from build123d import *

# Parameters (mm, degrees)
F2_START = 1.5
F0_W     = 68
F0_H     = 32
F0_W_2   = 66.0000007396
F0_H_2   = 30
F2_DEPTH = 4.5
F5_START = 0.9
F3_W     = 9.7086578608
F3_H     = 13.6771607213
F5_DEPTH = 2.3
F6_START = 1
F1_W     = 13.5039854795
F1_H     = 7.9890675843
F1_W_2   = 10.1785697043
F1_W_3   = 10.0000035018
F1_H_2   = 7.8571438789
F6_DEPTH = 4.6
F7_START = 1.5
F4_W     = 54.7266360372
F4_H     = 8.1930877641
F7_DEPTH = 4


with BuildPart() as f2:
    # F0 (on Top) → F2 (new body)
    with BuildSketch(Plane.XY.offset(F2_START)):
        with Locations((0, -0.0852976367)):
            Rectangle(F0_W, F0_H)
        with Locations((0, -0.0852976367)):
            Rectangle(F0_W_2, F0_H_2, mode=Mode.SUBTRACT)
    extrude(amount=F2_DEPTH)

    # F3 (on Top) → F5 (cut)
    with BuildSketch(Plane.XY.offset(F5_START)):
        with Locations((-30.4173231125, 1.8361529801)):
            Rectangle(F3_W, F3_H)
    extrude(amount=F5_DEPTH, mode=Mode.SUBTRACT)

    # F1 (on Top) → F6 (cut)
    with BuildSketch(Plane.XY.offset(F6_START)):
        with Locations((-19.5872941986, -13.5481059551)):
            Rectangle(F1_W, F1_H)
        with Locations((8.9285718277, -13.5481059551)):
            Rectangle(F1_W_2, F1_H)
        with Locations((21.8750005588, -13.4821441025)):
            Rectangle(F1_W_3, F1_H_2)
    extrude(amount=F6_DEPTH, mode=Mode.SUBTRACT)

    # F4 (on Top) → F7 (cut)
    with BuildSketch(Plane.XY.offset(F7_START)):
        with Locations((0.0114953145, 13.3686042391)):
            Rectangle(F4_W, F4_H)
    extrude(amount=F7_DEPTH, mode=Mode.SUBTRACT)


solid = f2.part
Read the model definition and answer for the solid it produces. Units are mm, in the model's axes. A direction names the side the tool comes from. Round coordinates to 2 decimals unless told otherwise and drop trailing zeros. Write each loop counter-clockwise with the first axis right and the second up, starting at its lowest first coordinate (ties: lowest second). Pieces come first, ordered by that corner, then holes.
1. The part is cut by section C-C, the plane z = 4.8. Determine the outline of the cut face in (x, y) (3 decimals).
2. Straight lines are drawn through the part: L1, parallel to X at y = 12.5, z = 5.35; L2, parallel to Y at x = 28, z = 3.85; L3, parallel to Y at x = -11, z = 1.95. For each, find the intervals that lie inside material, in ascending order.
3. The part is cut by section B-B, the plane y = -7. Determine the outline of the cut face in (x, z), then the cut area to 3 significant figures.
4. Which of the six approach directions +Z, -Z, +X, -X, +Y, -Y give full straight-line access (tool end or side, diameter ignored) to faces 4 (the face through (-33, 0, 4)), 5 (the face through (34, 0, 4))?
5. Given pin 1 Ø1.1 at (x, y) = (-21, -15.5) entering from -Z; pin 2 Ø10 at (x, y) = (-3, 5.5) entering from +Z; pin 3 Ø8 at (x, y) = (4.5, -12) entering from +Z; pin 4 Ø1.1 at (x, y) = (1.5, 15.5) entering from -Z, each flat-ended and moving along its own axis, determine where each tip first touches the part or whether it passes through.
6. The part is cut by section A-A, the plane x = -13.5. Determine the outline of the cut face in (y, z), then the cut area to 3 significant figures.
7. Determine the mould class of faces 1 (the face through (-33.2, 13.9, 1.5)), 2 (the face through (33, 0, 4)), 3 (the face through (0, -16.085, 4)) for opening direction Y: pulls with the +Y half, pulls with the -Y half, needs draft (parallel to the pull), parting line crosses it, or undercut.
Values:
1. outline: (-34, -16.085) - (-26.339, -16.085) - (-26.339, -15.085) - (-33, -15.085) - (-33, 14.915) - (-27.352, 14.915) - (-27.352, 15.915) - (-34, 15.915) - close; (-12.835, -16.085) - (3.839, -16.085) - (3.839, -15.085) - (-12.835, -15.085) - close; (14.018, -16.085) - (16.875, -16.085) - (16.875, -15.085) - (14.018, -15.085) - close; (26.875, -16.085) - (34, -16.085) - (34, 15.915) - (27.375, 15.915) - (27.375, 14.915) - (33, 14.915) - (33, -15.085) - (26.875, -15.085) - close
2. L1: x = -34 to -33, 33 to 34
2. L2: y = -16.09 to -15.09, 14.91 to 15.91
2. L3: y = -16.09 to -15.09
3. outline: (-34, 1.5) - (-33, 1.5) - (-33, 6) - (-34, 6) - close; (33, 1.5) - (34, 1.5) - (34, 6) - (33, 6) - close
3. area: 9.00 mm2
4. face 4: +Z, -Z
4. face 5: +Z, -Z, +X, +Y, -Y
5. pin 1: stops at z = 5.6
5. pin 2: passes through
5. pin 3: stops at z = 6
5. pin 4: stops at z = 5.5
6. outline: (-16.09, 5.6) - (-15.09, 5.6) - (-15.09, 6) - (-16.09, 6) - close; (14.91, 5.5) - (15.91, 5.5) - (15.91, 6) - (14.91, 6) - close
6. area: 0.900 mm2
7. face 1: needs draft
7. face 2: undercut
7. face 3: pulls with the -Y half
